from build123d import *

# Parameters (mm, degrees)
BOSS_EXTRUDE1_DEPTH = 18.5
SKETCH3_R           = 5.925
BOSS_EXTRUDE2_DEPTH = 10
SKETCH5_W           = 13.896314966
SKETCH5_H           = 3.370486285
CUT_EXTRUDE2_DEPTH  = 46.255082587
CHAMFER1_SIZE       = 1.5
CHAMFER1_SIZE2      = 0.401923789
CUT_EXTRUDE4_REACH  = 35.282
SKETCH7_W           = 8.5
SKETCH7_H           = 1.15
SKETCH9_W           = 14.675
SKETCH9_H           = 1.5
BOSS_EXTRUDE5_DEPTH = 1.8
FILLET8_R           = 1.5
SKETCH10_W          = 2.675
SKETCH10_H          = 1.5
BOSS_EXTRUDE6_DEPTH = 0.875
FILLET9_R           = 10
FILLET10_R          = 10


# Some blends are built 0.0001 mm under size
with BuildPart() as part:
    # Sketch2 → Boss-Extrude1 (new, symmetric)
    with BuildSketch(Plane(origin=(0, 0, 0), x_dir=(1, 0, 0), z_dir=(0, 1, 0))):
        Polygon((12, 3.25), (0, 3.25), (0, -3.25), (25, -3.25), (25, -5.925), (-2.675, -5.925), (-2.675, 5.925), (12, 5.925), align=None)
    extrude(amount=BOSS_EXTRUDE1_DEPTH, both=True)

    # Sketch3 → Boss-Extrude2 (add)
    with BuildSketch(Plane.ZY.offset(2.675)):
        with Locations(Location((1.425, 0, 0), (0, 0, 319.419581344))):
            Circle(SKETCH3_R)
    extrude(amount=BOSS_EXTRUDE2_DEPTH)

    # Sketch5 → Cut-Extrude2 (cut, through all)
    with BuildSketch(Plane(origin=(0, 18.5, 0), x_dir=(1, 0, 0), z_dir=(0, 1, 0))):
        with Locations((-9.623157483, -7.610243143)):
            Rectangle(SKETCH5_W, SKETCH5_H)
    extrude(amount=-CUT_EXTRUDE2_DEPTH, mode=Mode.SUBTRACT)

    # Chamfer1
    chamfer1_edges = [part.edges().sort_by_distance(p)[0] for p in [
        (-12.675, 0, -4.5),
    ]]
    chamfer1_side = [part.faces().sort_by_distance(p)[0] for p in [
        (-7.675, 0, -4.5),
    ]]
    chamfer(chamfer1_edges, length=CHAMFER1_SIZE, length2=CHAMFER1_SIZE2, reference=chamfer1_side[0])

    # Sketch7 → Cut-Extrude4 (cut, up to next)
    with BuildSketch(Plane(origin=(0, 0, -5.925), x_dir=(-1, 0, 0), z_dir=(0, 0, -1)), mode=Mode.PRIVATE) as cut_extrude4_sk1:
        with Locations((-7.75, -17.925)):
            Rectangle(SKETCH7_W, SKETCH7_H)
    cut_extrude4_tool1 = extrude(cut_extrude4_sk1.sketch, amount=-CUT_EXTRUDE4_REACH, mode=Mode.PRIVATE) & part.part
    add(cut_extrude4_tool1.solids().sort_by_distance((7.75, -17.925, -5.925))[0], mode=Mode.SUBTRACT)

    # Sketch9 → Boss-Extrude5 (add)
    with BuildSketch(Plane.XY.offset(-3.25)):
        with Locations((4.6625, -19.25)):
            Rectangle(SKETCH9_W, SKETCH9_H)
        with BuildLine():
            Line((11, -17.35), (10, -17.35))
            ThreePointArc((10, -17.35), (10.5, -17.85), (11, -17.35))
        make_face()
    extrude(amount=-BOSS_EXTRUDE5_DEPTH)

    # Fillet8
    fillet8_edges = [part.edges().sort_by_distance(p)[0] for p in [
        (-1.3375, -18.5, -3.25),
    ]]
    fillet(fillet8_edges, radius=FILLET8_R - 0.0001)  # a hair under: the kernel refuses the full size

    # Sketch10 → Boss-Extrude6 (add)
    with BuildSketch(Plane(origin=(0, 0, -5.05), x_dir=(-1, 0, 0), z_dir=(0, 0, -1))):
        with Locations((1.3375, -19.25)):
            Rectangle(SKETCH10_W, SKETCH10_H)
    extrude(amount=BOSS_EXTRUDE6_DEPTH)

    # Fillet9
    # the kernel refuses this fillet: 10 mm, written as the material it adds along each edge
    with BuildSketch(Plane(origin=(0, -20, -5.05), x_dir=(1, 0, 0), z_dir=(0, 1, 0))) as fillet9_piece_1:
        with BuildLine():
            CenterArc((4.090767043, 10), FILLET9_R, 245.853152003, 24.146847997)
            Line((0, 0.875), (0, 0))
            Line((0, 0), (4.090767043, 0))
        make_face()
    extrude(amount=1.5)

    # Fillet10
    fillet10_edges = [part.edges().sort_by_distance(p)[0] for p in [
        (25, 18.5, 4.5875),
        (12, 18.5, -4.5875),
        (25, -18.5, 4.5875),
    ]]
    fillet(fillet10_edges, radius=FILLET10_R)


solid = part.part
Work out the finished part from the listing and answer in its coordinate system (mm). A direction names the side the tool comes from. Coordinates: 2 decimals unless noted, no trailing zeros. Write each loop counter-clockwise with the first axis right and the second up, starting at its lowest first coordinate (ties: lowest second). Pieces come first, ordered by that corner, then holes. Notation, with made-up numbers: M -14,-25 L -6,-25 A26 cw -6,-3 Z; hole C 46,15 d8. An arc over 180 degrees is marked long. Write item = value, one per line.
1. The part is cut by section D-D (y = 13). Determine the outline of the cut face in (x, z) (3 decimals).
Solution:
outline = M -2.675,-5.925 L 10.93,-5.925 L 10.93,-3.25 L 0,-3.25 L 0,3.25 L 23.93,3.25 L 23.93,5.925 L -2.675,5.925 Z
2. The part is cut by section C-C (x = 22.5). Determine the outline of the cut face in (y, z) (3 decimals), then the cut area to 3 significant figures.
Solution:
outline = M -15.114,3.25 L 15.114,3.25 L 15.114,5.925 L -15.114,5.925 Z
area = 80.9 mm2
3. Determine the mould class of faces 1 (the face through (4, 18.5, 4)), 2 (the face through (21.99, -15.65, 4.61)), 3 (the face through (10.49, -17.85, -4.14)) for opening direction Y: released by +Y, released by -Y, zero draft, split by the parting line, or undercut.
Solution:
face_1 = released by +Y
face_2 = released by -Y
face_3 = undercut
4. Straight lines are drawn through the part: line 1 (Z direction, x = 1, y = 3.5) (3 decimals); line 2 (X direction, y = 13, z = 1.25) (3 decimals); line 3 (Z direction, x = 22.5, y = -11) (3 decimals). For each, find the intervals that lie inside material, in ascending order. Write a range as from..to.
Solution:
line_1 = -5.925..-3.25, 3.25..5.925
line_2 = -2.675..0
line_3 = 3.25..5.925
5. For faces 4 (the face through (8, -17.35, -5)), 5 (the face through (-6.866, 0.202, -4.497)), 6 (the face through (0, 0, 0)), determine the directions among +Z, -Z, +X, -X, +Y, -Y from which every point of the face is accessible in a straight line to the end or side of a thin tool.
Solution:
face_4 = -Z
face_5 = -X
face_6 = +X, +Y, -Y
6. The part is cut by section B-B (x = 9). Determine the outline of the cut face in (y, z) (3 decimals), then the cut area to 3 significant figures.
Solution:
outline = M -20,-5.05 L -18.5,-5.05 L -18.5,-3.25 L -20,-3.25 Z; M -18.5,3.25 L 18.5,3.25 L 18.5,5.925 L -18.5,5.925 Z; M -17.35,-5.925 L 15.641,-5.925 L 15.641,-3.25 L -17.35,-3.25 Z
area = 190 mm2
7. The part is cut by section A-A (y = 0). Determine the outline of the cut face in (x, z) (3 decimals).
Solution:
outline = M -12.675,-4.098 L -11.175,-4.5 L -2.675,-4.5 L -2.675,-5.925 L 12,-5.925 L 12,-3.25 L 0,-3.25 L 0,3.25 L 25,3.25 L 25,5.925 L -12.675,5.925 Z
8. Flat-ended cylindrical pins translate along their axes: pin 1 (1.3 mm diameter, centred on y = -3.5, z = -4, fed in from +X); pin 2 (6 mm diameter, centred on y = 8, z = -3, fed in from -X) (3 decimals); pin 3 (1.5 mm diameter, centred on x = 6, z = -4, fed in from +Y). Find the tip coordinate at first contact, or state that the pin passes through.
Solution:
pin_1 = 12
pin_2 = -2.675
pin_3 = 17.96
